Input: part model. Units: mm. Frame: model coordinates. Give positions to 0.01 mm unless a question says otherwise; leave off trailing zeros. Order: outer loops, then holes, each group sorted by start corner. A loop starts at its lowest first (then second) coordinate and runs counter-clockwise, first axis right, second up. Notation, with made-up numbers: M 2,16 L 39,16 A22 ccw 39,25 Z; hole C 68.25,-25.75 d5. An arc over 180 degrees is marked long. Use a Markdown table: item, result.
from build123d import *

# Parameters (mm, degrees)
SKETCH1_W           = 54
SKETCH1_H           = 88
BOSS_EXTRUDE1_DEPTH = 1
BOSS_EXTRUDE2_DEPTH = 2
FILLET4_R           = 0.1
FILLET5_R           = 0.1


with BuildPart() as part:
    # Sketch1 → Boss-Extrude1 (new body)
    with BuildSketch(Plane(origin=(0, 0, 0), x_dir=(1, 0, 0), z_dir=(0, 1, 0))):
        Rectangle(SKETCH1_W, SKETCH1_H)
    extrude(amount=BOSS_EXTRUDE1_DEPTH)

    # Sketch2 → Boss-Extrude2 (add)
    with BuildSketch(Plane.XZ):
        Polygon((-4, 42.7), (4, 42.7), (4, 44), (4, 50), (-4, 50), (-4, 44), align=None)
    extrude(amount=BOSS_EXTRUDE2_DEPTH)

    # Fillet4
    fillet4_edges = [part.edges().sort_by_distance(p)[0] for p in [
        (0, 0, 44),
    ]]
    fillet(fillet4_edges, radius=FILLET4_R)

    # Fillet5
    fillet5_edges = [part.edges().sort_by_distance(p)[0] for p in [
        (-4, 0, 43.35),
        (0, 0, 42.7),
        (4, 0, 43.35),
    ]]
    fillet(fillet5_edges, radius=FILLET5_R)


solid = part.part
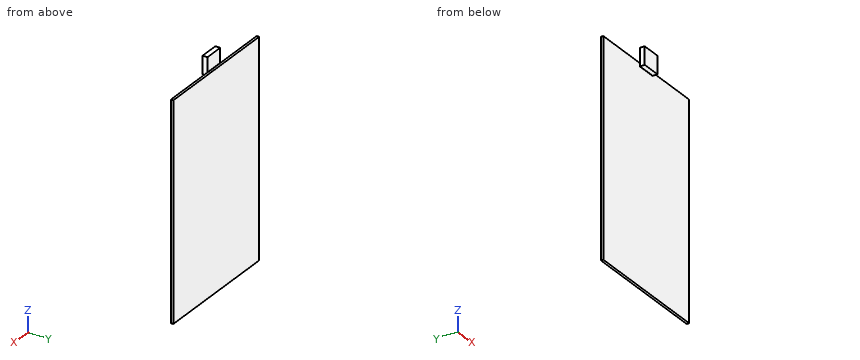
1) Material intervals for line 1 (Z direction, x = -18.5, y = 0.2); line 2 (Y direction, x = 18, z = -8); line 3 (Z direction, x = -3, y = -0.7), sorted ascending. Write a range as from..to.
Response values:
| item | result |
|---|---|
| line 1 | z = -44..44 |
| line 2 | y = 0..1 |
| line 3 | z = 42.7..50 |
2) Cut plane A-A on x = -0.5. Return loops of the section in (y, z).
Response values:
| item | result |
|---|---|
| outline | M -2,42.7 L -0.1,42.7 A0.1 cw 0,42.6 L 0,-44 L 1,-44 L 1,44 L 0.1,44 A0.1 cw 0,44.1 L 0,50 L -2,50 Z |
3) Cut plane B-B on z = -5.5. Return loops of the section in (x, y), and give its area (3 significant figures).
Response values:
| item | result |
|---|---|
| outline | M -27,0 L 27,0 L 27,1 L -27,1 Z |
| area | 54.0 mm² |
4) First-contact query: pin 1 Ø3 at (x, z) = (0, 47) entering from +Y; pin 2 Ø1 at (y, z) = (-0.5, 46) entering from -X; pin 3 Ø1.2 at (x, y) = (7, 0) entering from +Z. Flat tips, straight axial feed; report the tip coordinate or a pass-through.
Response values:
| item | result |
|---|---|
| pin 1 | stops at y = 0 |
| pin 2 | stops at x = -4 |
| pin 3 | stops at z = 44 |
5) Cut plane C-C on y = -1.25. Return loops of the section in (x, z).
Response values:
| item | result |
|---|---|
| outline | M -4,42.7 L 4,42.7 L 4,50 L -4,50 Z |
